Check sheet for the modelled part. Datum: model origin and axes. Units: mm. A direction names the side the tool comes from. Give positions to 0.01 mm unless a question says otherwise; leave off trailing zeros. Loops run counter-clockwise (first coordinate to the right, second up) from the corner with the lowest first, then second, coordinate; pieces in that order, holes last. Notation, with made-up numbers: M 59,-9.5 L 75,-9.5 A27 cw 75,16.5 Z; hole C 23,-15 d2. An arc over 180 degrees is marked long. Write each question's results on one line, items separated by ' | '. Start each with the question number.
1. Draft check along Y on faces 1 (the cylindrical face through (5.38, 31.01, 3.29)), 2 (the cylindrical face through (5.38, 3.29, -0.03)). Enter one of: pulls with the +Y half, pulls with the -Y half, needs draft (parallel to the pull), parting line crosses it, or undercut.
2. Material ranges on line 1 along Y through (x, z) = (5, -1); line 2 along Z through (x, y) = (-5, -30.85); line 3 along Y through (x, z) = (-0.75, 7.5), recorded low to high.
3. Sectioned sample at C-C on x = -0.5. Record the cut outline in (y, z).
4. Tool access check on faces 3 (the flat face through (0, -30, -6)), 4 (the flat face through (0, -30, 6)), 5 (the cylindrical face through (-3.25, -30.99, -4.92)). Record the directions out of +Z, -Z, +X, -X, +Y, -Y that give a thin tool (end or side, any length) a straight path to the whole face; none if there is none.
5. Go/stop test with a flat-tipped pin: pin 1 (10 mm diameter, centred on x = 1.5, y = 4, fed in from -Z). Record where the tip stops, or that it passes through.
6. Sectioned sample at B-B on z = -0.75. Give the number of separate pieces and of enclosed holes in the cut face, and give its area (3 significant figures).
7. Sectioned sample at D-D on y = 19. Record the cut outline in (x, z).
8. Sectioned sample at A-A on y = -5. Record the cut outline in (x, z).
```python
from build123d import *

# Parameters (mm, degrees)
F0_W     = 20
F0_H     = 60
F1_DEPTH = 2
F3_DEPTH = 2
F5_D     = 3.5
F6_W     = 20
F6_H     = 8
F6_H_2   = 4
F7_DEPTH = 2
F9_D     = 3.5
F10_R    = 5


# Not quite as in the source:
# - a feature names something its author has since deleted; it is built from what else it names


with BuildPart() as f1:
    # F0 (on Top) → F1 (new body, symmetric)
    with BuildSketch(Plane.XY):
        Rectangle(F0_W, F0_H)
    extrude(amount=F1_DEPTH, both=True)

    # F2 (on face) → F3 (join)
    with BuildSketch(Plane(origin=(0, 30, 0), x_dir=(-1, 0, 0), z_dir=(0, 1, 0))):
        Polygon((10, 2), (-2, 2), (2, -2), (10, -2), align=None)
        Polygon((-2, 2), (-10, 2), (-10, -2), (2, -2), align=None)
        Polygon((10, 10), (-10, 10), (-2, 2), (10, 2), align=None)
        Polygon((2, -2), (-10, -2), (-10, -10), (10, -10), align=None)
        Polygon((10, -2), (2, -2), (10, -10), align=None)
        Polygon((-2, 2), (-10, 10), (-10, 2), align=None)
    extrude(amount=F3_DEPTH)

    # F5 (through all)
    with Locations(Plane.XY.offset(2)):
        with Locations((5, 15), (-5, 15), (-5, 5), (5, 5), (5, -5), (-5, -5), (-5, -15), (5, -15)):
            Hole(F5_D / 2)

    # F6 (on face) → F7 (join)
    with BuildSketch(Plane.XZ.offset(30)):
        with Locations((0, 6)):
            Rectangle(F6_W, F6_H)
        Rectangle(F6_W, F6_H_2)
        with Locations((0, -6)):
            Rectangle(F6_W, F6_H)
    extrude(amount=F7_DEPTH)

    # F9 (through all)
    with Locations(Plane.XZ.offset(32)):
        with Locations((-5, 5), (5, 5), (5, -5), (-5, -5)):
            Hole(F9_D / 2)

    # F10
    f10_edges = [f1.edges().sort_by_distance(p)[0] for p in [
        (10, -31, 10),
        (10, -31, -10),
        (10, 31, 10),
        (10, 31, -10),
        (-10, 31, -10),
        (-10, 31, 10),
        (-10, -31, 10),
        (-10, -31, -10),
    ]]
    fillet(f10_edges, radius=F10_R)


solid = f1.part
```
Output values:
1) face 1: needs draft | face 2: undercut
2) line 1: -32 to -16.75, -13.25 to -6.75, -3.25 to 3.25, 6.75 to 13.25, 16.75 to 32 | line 2: -10 to -6.75, -3.25 to 3.25, 6.75 to 10 | line 3: -32 to -30, 30 to 32
3) outline: M -32,-10 L -30,-10 L -30,-2 L 30,-2 L 30,-10 L 32,-10 L 32,10 L 30,10 L 30,2 L -30,2 L -30,10 L -32,10 Z
4) face 3: -Z, +X, -X | face 4: +Z, +X, -X | face 5: +Y, -Y
5) pin 1: z = -2
6) separate pieces: 1 | enclosed holes: 8 | area: 1,200 mm2
7) outline: M -10,-2 L 10,-2 L 10,2 L -10,2 Z
8) outline: M -10,-2 L -6.75,-2 L -6.75,2 L -10,2 Z; M -3.25,-2 L 3.25,-2 L 3.25,2 L -3.25,2 Z; M 6.75,-2 L 10,-2 L 10,2 L 6.75,2 Z
